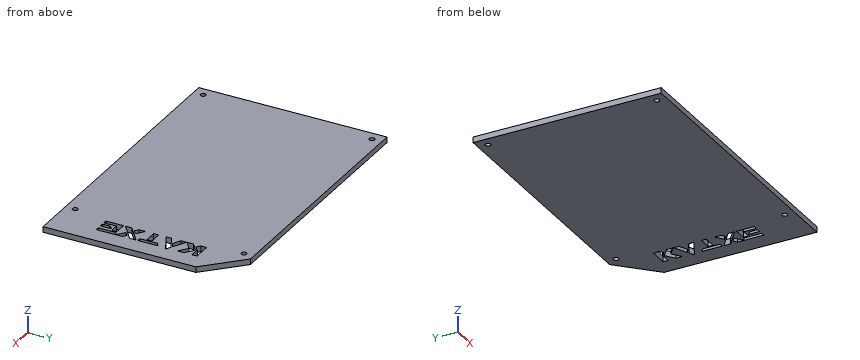
from build123d import *

# Parameters (mm, degrees)
SKETCH1_W           = 140.5
SKETCH1_H           = 106.5
SKETCH1_R           = 1.5
SKETCH1_W_2         = 2
BOSS_EXTRUDE1_DEPTH = 3.175
BOSS_EXTRUDE2_DEPTH = 3.175
SKETCH3_W           = 7.162162162
SKETCH3_H           = 2.850506757
CUT_EXTRUDE1_DEPTH  = 3.175


with BuildPart() as part:
    # Sketch1 → Boss-Extrude1 (new body)
    # profile 1 of 2: a face of its own
    with BuildSketch(Plane.XY):
        Rectangle(SKETCH1_W, SKETCH1_H)
        with Locations((-66.75, -47.75)):
            Circle(SKETCH1_R, mode=Mode.SUBTRACT)
        with Locations((66.75, -47.75)):
            Circle(SKETCH1_R, mode=Mode.SUBTRACT)
        with Locations((-66.75, 47.75)):
            Circle(SKETCH1_R, mode=Mode.SUBTRACT)
        with Locations((66.75, 47.75)):
            Circle(SKETCH1_R, mode=Mode.SUBTRACT)
    # profile 2 of 2: a face of its own
    with BuildSketch(Plane.XY):
        with Locations((-71.25, 0)):
            Rectangle(SKETCH1_W_2, SKETCH1_H)
    extrude(amount=BOSS_EXTRUDE1_DEPTH)

    # Sketch2 → Boss-Extrude2 (add)
    with BuildSketch(Plane.XY):
        Polygon((90.25, 33.25), (70.25, 53.25), (70.25, -53.25), (90.25, -53.25), align=None)
    extrude(amount=BOSS_EXTRUDE2_DEPTH)

    # Sketch3 → Cut-Extrude1 (cut)
    with BuildSketch(Plane.XY.offset(3.175)):
        Polygon((75.25, 21.279560811), (70.25, 17.358530405), (70.25, 21.064189189), (75.25, 24.985219595), (80.25, 21.064189189), (80.25, 17.358530405), align=None)
        Polygon((80.25, 28.475506757), (80.25, 25.625), (74.42652027, 25.625), (74.654560811, 25.447635135), (72.291807432, 23.595861486), (70.25, 25.19847973), (70.25, 28.475506757), align=None)
        Polygon((78.562922297, 12.801942568), (81.413429054, 11.326013514), (70.25, 5.553209459), (70.25, 8.616976351), align=None)
        Polygon((74.764358108, 11.746199324), (70.25, 14.032939189), (70.25, 17.098817568), (77.720439189, 13.234797297), align=None)
        Polygon((78.106841216, -5.014780405), (78.106841216, 4.961993243), (80.25, 6.387246622), (80.25, -5.014780405), align=None)
        with Locations((73.831081081, -0.025337837)):
            Rectangle(SKETCH3_W, SKETCH3_H)
        Polygon((70.25, -17.506334459), (70.25, -13.800675676), (80.25, -5.960726351), (80.25, -9.666385135), align=None)
        Polygon((78.208192568, -12.195945946), (80.25, -13.800675676), (80.25, -17.506334459), (75.843327703, -14.049831081), align=None)
        Polygon((72.291807432, -11.269003378), (70.25, -9.666385135), (70.25, -5.960726351), (74.654560811, -9.41722973), align=None)
        Polygon((78.106841216, -28.528293919), (78.106841216, -18.55152027), (80.25, -17.126266892), (80.25, -28.528293919), align=None)
        Polygon((77.376266892, -18.55152027), (77.376266892, -21.402027027), (72.393158784, -21.402027027), (72.393158784, -28.528293919), (70.25, -28.528293919), (70.25, -18.55152027), align=None)
        Polygon((73.782516892, -28.528293919), (73.782516892, -24.252533784), (75.925675676, -22.113597973), (75.925675676, -28.528293919), align=None)
    extrude(amount=-CUT_EXTRUDE1_DEPTH, mode=Mode.SUBTRACT)


solid = part.part
Model file for the job. Use its own axes, mm. Give positions to 0.01 mm unless a question says otherwise; leave off trailing zeros. Write each loop counter-clockwise with the first axis right and the second up, starting at its lowest first coordinate (ties: lowest second). Pieces come first, ordered by that corner, then holes. Notation, with made-up numbers: (17, 26.5) -> (23, 26.5) arc R24 ccw to (23, 53.5) -> close; hole circle Ø10 at (67, 14.25). An arc over 180 degrees is marked (long way). Write item = value, one per line.
(1) Flat gauge pin, fed straight in: P1, Ø0.6, axis at x = 79, z = 1.5, coming from the +Y side. Where does the tip first touch, or does it go through?
Determined:
P1 = 44.8
(2) Slice it at B-B, the plane z = 0.5. Give the number of separate pieces and of enclosed holes in the cut face, then the cut area to 3 significant figures.
Determined:
separate_pieces = 1
enclosed_holes = 15
area = 16,800 mm2
(3) Slice it at A-A, the plane y = 19. Give the cut face in (x, z) (3 decimals), then the cut area to 3 significant figures.
Determined:
outline = (-72.25, 0) -> (70.25, 0) -> (70.25, 3.175) -> (-72.25, 3.175) -> close; (72.343, 0) -> (78.157, 0) -> (78.157, 3.175) -> (72.343, 3.175) -> close; (80.25, 0) -> (90.25, 0) -> (90.25, 3.175) -> (80.25, 3.175) -> close
area = 503 mm2
(4) Probe line 1 along Y through (x, z) = (66.75, 2.25); line 2 along X through (y, z) = (-19.5, 2.5); line 3 along X through (y, z) = (-48, 1.45). List the from-to ranges inside material, lowest first.
Determined:
line_1 = -53.25 to -49.25, -46.25 to 46.25, 49.25 to 53.25
line_2 = -72.25 to 70.25, 77.38 to 78.11, 80.25 to 90.25
line_3 = -72.25 to -68.23, -65.27 to 65.27, 68.23 to 90.25
